Here's how the part is built. I have some questions about the finished solid (model axes, mm). A direction names the side the tool comes from. Round coordinates to 2 decimals unless told otherwise and drop trailing zeros. Loops run counter-clockwise (first coordinate to the right, second up) from the corner with the lowest first, then second, coordinate; pieces in that order, holes last. Notation, with made-up numbers: M -16.5,53.25 L 21.5,53.25 A22 cw 21.5,73.25 Z; hole C 59.25,34 d5. An arc over 180 degrees is marked long. Answer as a JSON object with one key per item and string values.
from build123d import *

# Parameters (mm, degrees)
SKETCH_2_W            = 210
SKETCH_2_H            = 100
EXTRUDE_1_DEPTH       = 4
SKETCH_7_R            = 3
CUT_EXTRUDE_2_DEPTH   = 1
SKETCH_8_R            = 3.1
CUT_EXTRUDE_3_DEPTH   = 60
SKETCH_11_OUTSIDE_W   = 258.526
SKETCH_11_OUTSIDE_H   = 148.526
SKETCH_11_OUTSIDE_W_2 = 130
SKETCH_11_OUTSIDE_H_2 = 100
SKETCH_11_OUTSIDE_R   = 3.1
CUT_EXTRUDE_5_DEPTH   = 100


with BuildPart() as part:
    # 草图2 → 凸台-拉伸1 (new body)
    with BuildSketch(Plane.XY):
        Rectangle(SKETCH_2_W, SKETCH_2_H)
    extrude(amount=EXTRUDE_1_DEPTH)

    # 草图7 → 切除-拉伸2 (cut)
    with BuildSketch(Plane.XY.offset(4)):
        with Locations((0, -17.737584897)):
            Circle(SKETCH_7_R)
    extrude(amount=-CUT_EXTRUDE_2_DEPTH, mode=Mode.SUBTRACT)

    # 草图8 → 切除-拉伸3 (cut)
    with BuildSketch(Plane.XY.offset(4)):
        with Locations((-55, 10)):
            Circle(SKETCH_8_R)
        with Locations((-55, 40)):
            Circle(SKETCH_8_R)
        with Locations((-55, -20)):
            Circle(SKETCH_8_R)
        with Locations((55, 40)):
            Circle(SKETCH_8_R)
        with Locations((55, 10)):
            Circle(SKETCH_8_R)
        with Locations((55, -20)):
            Circle(SKETCH_8_R)
    extrude(amount=-CUT_EXTRUDE_3_DEPTH, mode=Mode.SUBTRACT)

    # 草图11 outside → 切除-拉伸5 (cut)
    # profile 1 of 2: a face of its own
    with BuildSketch(Plane(origin=(0, 0, 0), x_dir=(-1, 0, 0), z_dir=(0, 0, -1))):
        Rectangle(SKETCH_11_OUTSIDE_W, SKETCH_11_OUTSIDE_H)
        Rectangle(SKETCH_11_OUTSIDE_W_2, SKETCH_11_OUTSIDE_H_2, mode=Mode.SUBTRACT)
    # profile 2 of 2: a face of its own
    with BuildSketch(Plane(origin=(0, 0, 0), x_dir=(-1, 0, 0), z_dir=(0, 0, -1))):
        with Locations(Location((55, 40, 0), (0, 0, 180))):
            Circle(SKETCH_11_OUTSIDE_R)
    extrude(amount=-CUT_EXTRUDE_5_DEPTH, mode=Mode.SUBTRACT)


solid = part.part
Item 1: If we mould it in two halves opening along Y, with no side actions, what happens to faces 3 (the face through (-1, 1, 0)), 4 (the face through (-52.136, 8.813, 2.028)), 5 (the face through (-1, 50, 2))? For each: pulls with the +Y half, pulls with the -Y half, needs draft (parallel to the pull), parting line crosses it, or undercut.
Resolved:
{"face 3": "needs draft", "face 4": "undercut", "face 5": "pulls with the +Y half"}
Item 2: I want a section at A-A, the plane x = -55. Please give me the cut outline in (y, z).
Resolved:
{"outline": "M -50,0 L -23.1,0 L -23.1,4 L -50,4 Z; M -16.9,0 L 6.9,0 L 6.9,4 L -16.9,4 Z; M 13.1,0 L 36.9,0 L 36.9,4 L 13.1,4 Z; M 43.1,0 L 50,0 L 50,4 L 43.1,4 Z"}
Item 3: On a 3-axis mill with a long thin cutter (end or side, diameter ignored), from which of +Z, -Z, +X, -X, +Y, -Y can I reach the whole of each face in a straight line? I mean faces 1 (the face through (0, -18, 3)), 2 (the face through (57.864, 8.813, 2.028)). Say none if no direction works.
Resolved:
{"face 1": "+Z", "face 2": "+Z, -Z"}
Item 4: Please list where these lines run through material, in increasing order: probe 1 along Y at (x, z) = (-55, 3.15); probe 2 along X at (y, z) = (9, 3.5); probe 3 along X at (y, z) = (38, 1.85). Write a range as from..to.
Resolved:
{"probe 1": "-50..-23.1, -16.9..6.9, 13.1..36.9, 43.1..50", "probe 2": "-65..-57.93, -52.07..52.07, 57.93..65", "probe 3": "-65..-57.37, -52.63..52.63, 57.37..65"}
Item 5: I want a section at B-B, the plane y = 10. Please give me the cut outline in (x, z).
Resolved:
{"outline": "M -65,0 L -58.1,0 L -58.1,4 L -65,4 Z; M -51.9,0 L 51.9,0 L 51.9,4 L -51.9,4 Z; M 58.1,0 L 65,0 L 65,4 L 58.1,4 Z"}
Item 6: I want a section at C-C, the plane x = 0. Please give me the cut outline in (y, z).
Resolved:
{"outline": "M -50,0 L 50,0 L 50,4 L -14.74,4 L -14.74,3 L -20.74,3 L -20.74,4 L -50,4 Z"}
